```python
from build123d import *

# Parameters (mm, degrees)
BOSS_EXTRUDE1_DEPTH     = 38.1
CUT_EXTRUDE_THIN5_DEPTH = 35.814
CUT_EXTRUDE9_DEPTH      = 198.640484432
CUT_EXTRUDE9_DEPTH_BACK = 35.814
CUT_EXTRUDE10_DEPTH     = 7.62


with BuildPart() as part:
    # Sketch1 → Boss-Extrude1 (new body)
    with BuildSketch(Plane(origin=(0, 0, 0), x_dir=(1, 0, 0), z_dir=(0, 1, 0))):
        with BuildLine():
            Line((0, 11.43), (0, -11.43))
            Line((0, -11.43), (35.052, -5.249386672))
            Line((35.052, -5.249386672), (35.052, -19.981386672))
            Line((35.052, -19.981386672), (136.652, -19.981386672))
            Line((136.652, -19.981386672), (136.652, -70.781386672))
            ThreePointArc((136.652, -70.781386672), (154.559, -88.688386672), (172.466, -70.781386672))
            Line((172.466, -70.781386672), (172.466, 70.781386672))
            ThreePointArc((172.466, 70.781386672), (154.559, 88.688386672), (136.652, 70.781386672))
            Line((136.652, 70.781386672), (136.652, 19.981386672))
            Line((136.652, 19.981386672), (35.052, 19.981386672))
            Line((35.052, 19.981386672), (35.052, 5.249386672))
            Line((35.052, 5.249386672), (0, 11.43))
        make_face()
    extrude(amount=BOSS_EXTRUDE1_DEPTH)

    # Sketch3 → Cut-Extrude-Thin5 (cut)
    with BuildSketch(Plane(origin=(172.466, 0, 0), x_dir=(0, 0, -1), z_dir=(1, 0, 0))):
        Polygon((-40.668819045, 38.1), (-88.688386672, 24.903727481), (-102.149697549, 73.887736193), (-54.130129922, 87.084008712), align=None)
    extrude(amount=-CUT_EXTRUDE_THIN5_DEPTH, mode=Mode.SUBTRACT)

    # Sketch4 → Cut-Extrude9 (cut, two sides: drawn at the far end of the back side and taken through both)
    with BuildSketch(Plane(origin=(172.466, 0, 0), x_dir=(0, 0, -1), z_dir=(1, 0, 0)).offset(-CUT_EXTRUDE9_DEPTH_BACK)):
        Polygon((-314.400611186, 135.676742064), (40.668819045, 38.1), (88.688386672, 24.903727481), (443.757816904, -72.673014582), (638.911301031, 637.465845881), (-119.247127059, 845.815602527), align=None)
    extrude(amount=CUT_EXTRUDE9_DEPTH + CUT_EXTRUDE9_DEPTH_BACK, mode=Mode.SUBTRACT)

    # Sketch5 → Cut-Extrude10 (cut)
    with BuildSketch(Plane(origin=(0, 38.1, 0), x_dir=(1, 0, 0), z_dir=(0, 1, 0))):
        Polygon((0, -11.43), (0, 11.43), (0.210478784, 11.603037745), (35.052, 5.249386672), (35.052, -5.249386672), align=None)
    extrude(amount=-CUT_EXTRUDE10_DEPTH, mode=Mode.SUBTRACT)


solid = part.part
```
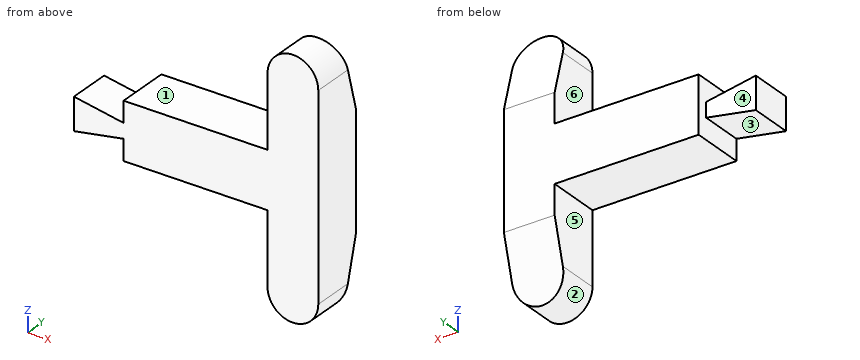
Check sheet for the modelled part. Datum: model origin and axes. Units: mm. Face numbers are marked on the shaded views. A direction names the side the tool comes from. Give positions to 0.01 mm unless a question says otherwise; leave off trailing zeros. Order: outer loops, then holes, each group sorted by start corner. A loop starts at its lowest first (then second) coordinate and runs counter-clockwise, first axis right, second up. Notation, with made-up numbers: (87, -36) -> (129, -36) arc R13 cw to (129, -11) -> close; hole circle Ø6 at (20.5, -30.75). An arc over 180 degrees is marked (long way). Return JSON: item names as keys, results as strings.
1. Cross-section at B-B, the plane x = 96.5. Record the cut outline in (y, z), plus the area to 3 significant figures.
From the geometry:
{"outline": "(0, -19.98) -> (38.1, -19.98) -> (38.1, 19.98) -> (0, 19.98) -> close", "area": "1,520 mm^2"}
2. Mould release check, pull along X, two halves, no side actions. Record for the marked faces 1, 2 and 3: +X half, -X half, draft (parallel to the pull), parting line (faces both ways), or undercut.
From the geometry:
{"face 1": "draft", "face 2": "parting line", "face 3": "undercut"}
3. Cross-section at D-D, the plane y = 34.5. Record the cut outline in (x, z), plus the area to 3 significant figures.
From the geometry:
{"outline": "(35.05, -19.98) -> (136.65, -19.98) -> (136.65, -53.77) -> (172.47, -53.77) -> (172.47, 53.77) -> (136.65, 53.77) -> (136.65, 19.98) -> (35.05, 19.98) -> close", "area": "7,910 mm^2"}
4. Cross-section at C-C, the plane z = -74.5. Record the cut outline in (x, y).
From the geometry:
{"outline": "(137.04, 0) -> (172.08, 0) -> (172.08, 28.8) -> (137.04, 28.8) -> close"}
5. Cross-section at A-A, the plane y = 17.5. Record the cut outline in (x, z), plus the area to 3 significant figures.
From the geometry:
{"outline": "(0, -11.43) -> (35.05, -5.25) -> (35.05, -19.98) -> (136.65, -19.98) -> (136.65, -70.78) arc R17.91 ccw to (172.47, -70.78) -> (172.47, 70.78) arc R17.91 ccw to (136.65, 70.78) -> (136.65, 19.98) -> (35.05, 19.98) -> (35.05, 5.25) -> (0, 11.43) -> close", "area": "10,700 mm^2"}
6. Go/stop test with flat-tipped pins: P1, Ø6, axis at y = 19.5, z = 32.5, coming from the -X side; P2, Ø1, axis at x = 137.5, y = 19.5, coming from the -Z side; P3, Ø18.5, axis at x = 22.5, z = -3.5, coming from the +Y side; P4, Ø6, axis at x = 122, z = 23.5, coming from the -Y side. Record where each tip stops, or that it passes through.
From the geometry:
{"P1": "x = 136.65", "P2": "z = -77.6", "P3": "y = 30.48", "P4": "through"}
7. Set-up check for the marked faces 4, 5 and 6: record each of +Z, -Z, +X, -X, +Y, -Y from which the full face is reachable in a straight line by a thin tool's end or side.
From the geometry:
{"face 4": "+Z, -Z, -X, +Y", "face 5": "-Z, -X, +Y, -Y", "face 6": "+Z, -X, +Y, -Y"}
8. Material ranges on probe 1 along X at (y, z) = (6, 30.5); probe 2 along X at (y, z) = (36.5, 14); probe 3 along Z at (x, y) = (135, 32), recorded low to high. Write a range as [from, to].
From the geometry:
{"probe 1": "[136.65, 172.47]", "probe 2": "[35.05, 172.47]", "probe 3": "[-19.98, 19.98]"}
